Here's how the part is built. I have some questions about the finished solid (model axes, mm). A direction names the side the tool comes from. Coordinates: 2 decimals unless noted, no trailing zeros. Write each loop counter-clockwise with the first axis right and the second up, starting at its lowest first coordinate (ties: lowest second). Pieces come first, ordered by that corner, then holes. Notation, with made-up numbers: (0.25, 46.25) -> (33.25, 46.25) arc R28 ccw to (33.25, 72.25) -> close; hole circle Ø5 at (45, 36.5). An arc over 180 degrees is marked (long way). Put each result on its own line as item: value.
Autodesk Inventor part; units mm, degrees
ref_plane "YZ Plane" through (0, 0, 0) normal (1, 0, 0) x (0, 1, 0)
ref_plane "XZ Plane" through (0, 0, 0) normal (0, 1, 0) x (-1, 0, 0)
ref_plane "XY Plane" through (0, 0, 0) normal (0, 0, 1) x (1, 0, 0)
sketch "Sketch1" plane through (0, 0, 0) normal (0, 0, 1) x (1, 0, 0)
  line L0 (11.43, -11.43) -> (-11.43, -11.43)
  line L1 (-11.43, -11.43) -> (-11.43, 11.43)
  line L2 (-11.43, 11.43) -> (11.43, 11.43)
  line L3 (11.43, 11.43) -> (11.43, -11.43)
  line L4 (11.43, -11.43) -> (-11.43, 11.43) construction
  line L5 (-11.43, -11.43) -> (11.43, 11.43) construction
  circle A0 centre (-8.89, 8.89) radius 1.27
  circle A1 centre (8.89, 8.89) radius 1.27
  line L6 (0, 11.43) -> (0, -11.43) construction
  circle A2 centre (-8.89, -8.89) radius 0.762
  circle A3 centre (-6.35, -8.89) radius 0.762
  circle A4 centre (-3.81, -8.89) radius 0.762
  circle A5 centre (-1.27, -8.89) radius 0.762
  circle A6 centre (1.27, -8.89) radius 0.762
  circle A7 centre (3.81, -8.89) radius 0.762
  circle A8 centre (6.35, -8.89) radius 0.762
  circle A9 centre (8.89, -8.89) radius 0.762
  point P0 (0, 0)
  dimension "d0" = 22.86
  dimension "d1" = 22.86
  dimension "d2" = 2.54
  dimension "d3" = 17.78
  dimension "d4" = 20.32
  dimension "d5" = 1.524
  dimension "d6" = 2.54
  dimension "d9" = 2.54
extrude "Extrusion1" add sketch "Sketch1" along normal blind 1.6
fillet "Fillet1" radius 2 4 edges at (-11.43, 11.43, 0.8) (11.43, 11.43, 0.8) (11.43, -11.43, 0.8) (-11.43, -11.43, 0.8)
sketch "Sketch2" plane through (0, 0, 1.6) normal (0, 0, 1) x (1, 0, 0)
  line L0 (2.25, -3.68) -> (-2.25, -3.68)
  line L1 (-2.25, -3.68) -> (-2.25, 1.32)
  line L2 (-2.25, 1.32) -> (2.25, 1.32)
  line L3 (2.25, 1.32) -> (2.25, -3.68)
  line L4 (2.25, -3.68) -> (-2.25, 1.32) construction
  line L5 (-2.25, -3.68) -> (2.25, 1.32) construction
  line L6 (9.43, 11.43) -> (-9.43, 11.43)
  line L7 (-9.43, -11.43) -> (9.43, -11.43)
  point P0 (0, 0)
  point P1 (0, -1.18)
  point P2 (0, -1.18)
  dimension "d17" = 4.5
  dimension "d18" = 5
  dimension "d20" = 12.75
extrude "Extrusion2" add sketch "Sketch2" along normal blind 1
chamfer "Chamfer1" distance 0.2 angle 45 2 edges at (-2.25, -1.18, 2.6) (2.25, -1.18, 2.6)
sketch "Sketch5" plane through (0, 0, 1.6) normal (0, 0, 1) x (1, 0, 0)
  line L0 (-11.3283, 11.4877) -> (11.6389, 11.4877) construction
  line L1 (11.6389, 11.4877) -> (11.6389, -11.3452) construction
  line L2 (11.6389, -11.3452) -> (-11.3283, -11.3452) construction
  line L3 (-11.3283, -11.3452) -> (-11.3283, 11.4877) construction
  point P0 (0, 0)
properties part number "Adafruit_INA260"
Item 1: Imagine slicing it at D-D on x = -8.89. Write out the boundary of the cut face in (y, z).
Output:
outline: (-11.43, 0) -> (-9.65, 0) -> (-9.65, 1.6) -> (-11.43, 1.6) -> close; (-8.13, 0) -> (7.62, 0) -> (7.62, 1.6) -> (-8.13, 1.6) -> close; (10.16, 0) -> (11.43, 0) -> (11.43, 1.6) -> (10.16, 1.6) -> close
Item 2: Imagine slicing it at C-C on y = 0.5. Write out the boundary of the cut face in (x, z), then the cut area to 3 significant figures.
Output:
outline: (-11.43, 0) -> (11.43, 0) -> (11.43, 1.6) -> (2.25, 1.6) -> (2.25, 2.4) -> (2.05, 2.6) -> (-2.05, 2.6) -> (-2.25, 2.4) -> (-2.25, 1.6) -> (-11.43, 1.6) -> close
area: 41.0 mm²
Item 3: For P1, Ø2.5, axis at x = 3.81, y = -8.89, coming from the +Z side; P2, Ø2, axis at x = 8.89, y = 8.89, coming from the -Z side (3 decimals), each with a flat end and sliding along its axis, tell me the tip position at first contact or that it passes through.
Output:
P1: stops at z = 1.6
P2: passes through
Item 4: If we mould it in two halves opening along X, with no side actions, what happens to faces 4 (the flat face through (0, -11.43, 1)), 5 (the cylindrical face through (-10.83, 10.86, 0.81)), 6 (the cylindrical face through (-9.452, -9.405, 0.789))? For each: released by +X, released by -X, zero draft, split by the parting line, or undercut.
Output:
face 4: zero draft
face 5: released by -X
face 6: undercut
Item 5: Imagine slicing it at B-B on z = 0.75. State how many separate pieces and enclosed holes the cut face has, then the cut area to 3 significant figures.
Output:
separate pieces: 1
enclosed holes: 10
area: 494 mm²
Item 6: Which directions (+Z, -Z, +X, -X, +Y, -Y) give clear straight access to the entire face, cutting with the end or side of a thin tool? Please do faces 1 (the cylindrical face through (8.328, -9.405, 0.789)), 2 (the flat face through (0, -3.68, 2)), 3 (the flat face through (0, 1.32, 2)).
Output:
face 1: +Z, -Z
face 2: +Z, +X, -X, -Y
face 3: +Z, +X, -X, +Y
Item 7: Please list where these lines run through material, in increasing order: line 1 along Y through (x, z) = (-8.89, 1.25); line 2 along Y through (x, z) = (-9.5, 1.1); line 3 along X through (y, z) = (8.75, 0.7). Write a range as from..to.
Output:
line 1: y = -11.43..-9.65, -8.13..7.62, 10.16..11.43
line 2: y = -11.43..-9.35, -8.43..7.78, 10..11.43
line 3: x = -11.43..-10.15, -7.63..7.63, 10.15..11.43
Item 8: Imagine slicing it at A-A on x = -6.35. Write out the boundary of the cut face in (y, z).
Output:
outline: (-11.43, 0) -> (-9.65, 0) -> (-9.65, 1.6) -> (-11.43, 1.6) -> close; (-8.13, 0) -> (11.43, 0) -> (11.43, 1.6) -> (-8.13, 1.6) -> close
